```python
from build123d import *

# Parameters (mm, degrees)
BOSS_EXTRUDE1_DEPTH = 317.5
SKETCH2_R           = 6.35
CUT_EXTRUDE1_DEPTH  = 304.8
FILLET1_R           = 2.54


with BuildPart() as part:
    # Sketch1 → Boss-Extrude1 (new body)
    with BuildSketch(Plane(origin=(0, 0, 0), x_dir=(1, 0, 0), z_dir=(0, 1, 0))):
        Polygon((0, 0), (50.8, 0), (50.8, 38.1), (41.275, 38.1), (41.275, 9.525), (9.525, 9.525), (9.525, 38.1), (0, 38.1), align=None)
    extrude(amount=BOSS_EXTRUDE1_DEPTH)

    # Sketch2 → Cut-Extrude1 (cut)
    with BuildSketch(Plane(origin=(50.8, 0, 0), x_dir=(0, 0, -1), z_dir=(1, 0, 0))):
        with Locations((22.86, 304.8)):
            Circle(SKETCH2_R)
        with Locations((22.86, 190.5)):
            Circle(SKETCH2_R)
        with Locations((22.86, 228.6)):
            Circle(SKETCH2_R)
        with Locations((22.86, 266.7)):
            Circle(SKETCH2_R)
        with Locations((22.86, 76.2)):
            Circle(SKETCH2_R)
        with Locations((22.86, 38.1)):
            Circle(SKETCH2_R)
        with Locations((22.86, 152.4)):
            Circle(SKETCH2_R)
        with Locations((22.86, 114.3)):
            Circle(SKETCH2_R)
    extrude(amount=-CUT_EXTRUDE1_DEPTH, mode=Mode.SUBTRACT)

    # Fillet1
    fillet1_edges = [part.edges().sort_by_distance(p)[0] for p in [
        (41.275, 158.75, -38.1),
        (9.525, 158.75, -38.1),
        (9.525, 158.75, -9.525),
        (41.275, 158.75, -9.525),
    ]]
    fillet(fillet1_edges, radius=FILLET1_R)


solid = part.part
```
Geometry: final body of the model. Coordinates: model frame, mm. A direction names the side the tool comes from. Coordinates: 2 decimals unless noted, no trailing zeros. Loops run counter-clockwise (first coordinate to the right, second up) from the corner with the lowest first, then second, coordinate; pieces in that order, holes last. Notation, with made-up numbers: M 55.5,77.25 L 73.5,77.25 A20 ccw 73.5,115.25 Z; hole C 39.25,-26 d3. An arc over 180 degrees is marked long. Put each result on its own line as item: value.
(1) Access query for faces 4 (the face through (41.275, 157, -29)), 5 (the face through (4, 157, -38.1)). Directions: +Z, -Z, +X, -X, +Y, -Y. A direction counts if a zero-diameter tool reaches every point of the face in a straight line with its end or side. Return the directions, or none.
Answer sheet:
face 4: -Z, +Y, -Y
face 5: -Z, +X, -X, +Y, -Y
(2) Cut plane B-B on z = -22.86. State how many separate pieces and enclosed holes the cut face has, then the cut area to 3 significant figures.
Answer sheet:
separate pieces: 18
enclosed holes: 0
area: 4,110 mm^2
(3) Cut plane A-A on y = 190.5. Return the cut outline in (x, z) (3 decimals), then the cut area to 3 significant figures.
Answer sheet:
outline: M 0,-38.1 L 6.985,-38.1 A2.54 ccw 9.525,-35.56 L 9.525,-29.21 L 0,-29.21 Z; M 0,-16.51 L 9.525,-16.51 L 9.525,-12.065 A2.54 cw 12.065,-9.525 L 38.735,-9.525 A2.54 cw 41.275,-12.065 L 41.275,-16.51 L 50.8,-16.51 L 50.8,0 L 0,0 Z; M 41.275,-35.56 A2.54 ccw 43.815,-38.1 L 50.8,-38.1 L 50.8,-29.21 L 41.275,-29.21 Z
area: 786 mm^2
(4) Material intervals for probe 1 along X at (y, z) = (158, -14.5) (3 decimals); probe 2 along Z at (x, y) = (26.5, 296) (3 decimals); probe 3 along Z at (x, y) = (45, 196), sorted ascending.
Answer sheet:
probe 1: x = 0 to 9.525, 41.275 to 50.8
probe 2: z = -9.525 to 0
probe 3: z = -38.1 to -26.03, -19.69 to 0
(5) Draft query along Z for faces 1 (the face through (25, 157, 0)), 2 (the face through (4.829, 196.796, -22.033)), 3 (the face through (9.525, 157, -29)). Return one class per face: pulls with the +Z half, pulls with the -Z half, needs draft (parallel to the pull), parting line crosses it, or undercut.
Answer sheet:
face 1: pulls with the +Z half
face 2: undercut
face 3: needs draft
(6) First-contact query: pin 1 (13.5 mm diameter, centred on x = 22.5, y = 95.5, fed in from -Z) (3 decimals). Flat tip, straight axial feed; report the tip coordinate or a pass-through.
Answer sheet:
pin 1: stops at z = -9.525
(7) Cut plane C-C on x = 35. Return the cut outline in (y, z) (3 decimals), then the cut area to 3 significant figures.
Answer sheet:
outline: M 0,-9.525 L 317.5,-9.525 L 317.5,0 L 0,0 Z
area: 3,020 mm^2
